Part model, mm, in its own coordinate system. A direction names the side the tool comes from. Give positions to 0.01 mm unless a question says otherwise; leave off trailing zeros. Loops run counter-clockwise (first coordinate to the right, second up) from the corner with the lowest first, then second, coordinate; pieces in that order, holes last. Notation, with made-up numbers: (-6, 50) -> (7, 50) arc R17 ccw to (7, 57) -> close; hole circle Ø9 at (-5.75, -27.75). An arc over 180 degrees is marked (long way). Write item = value, one per line.
from build123d import *

# Parameters (mm, degrees)
SKETCH1_W               = 12
SKETCH1_H               = 12
SKETCH1_R               = 5.5
BOSS_EXTRUDE1_DEPTH     = 6
BOSS_EXTRUDE1_2_DEPTH   = 6
BOSS_EXTRUDE1_3_DEPTH   = 6
BOSS_EXTRUDE1_4_DEPTH   = 6
BOSS_EXTRUDE1_5_DEPTH   = 6
BOSS_EXTRUDE1_6_DEPTH   = 6
BOSS_EXTRUDE2_START     = -6
BOSS_EXTRUDE2_OUTLINE_R = 1.7
BOSS_EXTRUDE2_DEPTH     = 6
CUT_EXTRUDE1_DEPTH      = 1


# Read off the part's stored shape, not the designer's step: Boss-Extrude2
with BuildPart() as part:
    # Sketch1 → Boss-Extrude1 (new body)
    with BuildSketch(Plane(origin=(0, 0, 0), x_dir=(1, 0, 0), z_dir=(0, 1, 0))):
        with Locations((13.686388819, -10.664882883)):
            Rectangle(SKETCH1_W, SKETCH1_H)
        with Locations(Location((13.686388819, -10.664882883, 0), (0, 0, 270))):
            Circle(SKETCH1_R, mode=Mode.SUBTRACT)
    extrude(amount=-BOSS_EXTRUDE1_DEPTH)



with BuildPart() as body_2:
    # Sketch1 → Boss-Extrude1 2 (new body)
    with BuildSketch(Plane(origin=(0, 0, 0), x_dir=(1, 0, 0), z_dir=(0, 1, 0))):
        with Locations((-1.113611181, -10.664882883)):
            Rectangle(SKETCH1_W, SKETCH1_H)
        with Locations(Location((-1.113611181, -10.664882883, 0), (0, 0, 270))):
            Circle(SKETCH1_R, mode=Mode.SUBTRACT)
    extrude(amount=-BOSS_EXTRUDE1_2_DEPTH)


with BuildPart() as body_3:
    # Sketch1 → Boss-Extrude1 3 (new body)
    with BuildSketch(Plane(origin=(0, 0, 0), x_dir=(1, 0, 0), z_dir=(0, 1, 0))):
        with Locations((6.28638882, -23.664882883)):
            Rectangle(SKETCH1_W, SKETCH1_H)
        with Locations(Location((6.28638882, -23.664882883, 0), (0, 0, 270))):
            Circle(SKETCH1_R, mode=Mode.SUBTRACT)
    extrude(amount=-BOSS_EXTRUDE1_3_DEPTH)


with BuildPart() as body_4:
    # Sketch1 → Boss-Extrude1 4 (new body)
    with BuildSketch(Plane(origin=(0, 0, 0), x_dir=(1, 0, 0), z_dir=(0, 1, 0))):
        with Locations((21.08638882, -23.664882883)):
            Rectangle(SKETCH1_W, SKETCH1_H)
        with Locations(Location((21.08638882, -23.664882883, 0), (0, 0, 270))):
            Circle(SKETCH1_R, mode=Mode.SUBTRACT)
    extrude(amount=-BOSS_EXTRUDE1_4_DEPTH)


with BuildPart() as body_5:
    # Sketch1 → Boss-Extrude1 5 (new body)
    with BuildSketch(Plane(origin=(0, 0, 0), x_dir=(1, 0, 0), z_dir=(0, 1, 0))):
        with Locations((35.88638882, -23.664882883)):
            Rectangle(SKETCH1_W, SKETCH1_H)
        with Locations(Location((35.88638882, -23.664882883, 0), (0, 0, 270))):
            Circle(SKETCH1_R, mode=Mode.SUBTRACT)
    extrude(amount=-BOSS_EXTRUDE1_5_DEPTH)


with BuildPart() as body_6:
    # Sketch1 → Boss-Extrude1 6 (new body)
    with BuildSketch(Plane(origin=(0, 0, 0), x_dir=(1, 0, 0), z_dir=(0, 1, 0))):
        with Locations((28.486388819, -10.664882883)):
            Rectangle(SKETCH1_W, SKETCH1_H)
        with Locations(Location((28.486388819, -10.664882883, 0), (0, 0, 270))):
            Circle(SKETCH1_R, mode=Mode.SUBTRACT)
    extrude(amount=-BOSS_EXTRUDE1_6_DEPTH)


with BuildPart() as part_1:
    add(part.part)

    add(body_2.part)  # Boss-Extrude2 merges body 2

    add(body_3.part)  # Boss-Extrude2 merges body 3

    add(body_4.part)  # Boss-Extrude2 merges body 4

    add(body_5.part)  # Boss-Extrude2 merges body 5

    add(body_6.part)  # Boss-Extrude2 merges body 6
    # Boss-Extrude2 outline → Boss-Extrude2 (add)
    with BuildSketch(Plane(origin=(0, 0, 0), x_dir=(1, 0, 0), z_dir=(0, 1, 0)).offset(BOSS_EXTRUDE2_START)):
        Polygon((11.186388819, -4.164882883), (1.386388819, -4.164882883), (1.386388819, -4.664882883), (4.886388819, -4.664882883), (4.886388819, -16.664882883), (-7.113611181, -16.664882883), (-7.113611181, -4.664882883), (-3.613611181, -4.664882883), (-3.613611181, -4.164882883), (-18.613611181, -4.164883527), (-18.613611181, -30.164882449), (3.78638882, -30.164882883), (3.78638882, -29.664882883), (0.28638882, -29.664882883), (0.28638882, -17.664882883), (12.28638882, -17.664882883), (12.28638882, -29.664882883), (8.78638882, -29.664882883), (8.78638882, -30.164882883), (18.58638882, -30.164882883), (18.58638882, -29.664882883), (15.08638882, -29.664882883), (15.08638882, -17.664882883), (27.08638882, -17.664882883), (27.08638882, -29.664882883), (23.58638882, -29.664882883), (23.58638882, -30.164882883), (33.38638882, -30.164882883), (33.38638882, -29.664882883), (29.88638882, -29.664882883), (29.88638882, -17.664882883), (41.88638882, -17.664882883), (41.88638882, -29.664882883), (38.38638882, -29.664882883), (38.38638882, -30.164882883), (53.38638882, -30.164882883), (53.38638882, -4.164882883), (30.986388819, -4.164882883), (30.986388819, -4.664882883), (34.486388819, -4.664882883), (34.486388819, -16.664882883), (22.486388819, -16.664882883), (22.486388819, -4.664882883), (25.986388819, -4.664882883), (25.986388819, -4.164882883), (16.186388819, -4.164882883), (16.186388819, -4.664882883), (19.686388819, -4.664882883), (19.686388819, -16.664882883), (7.686388819, -16.664882883), (7.686388819, -4.664882883), (11.186388819, -4.664882883), align=None)
        with Locations((-13.613611181, -17.164882988)):
            Circle(BOSS_EXTRUDE2_OUTLINE_R, mode=Mode.SUBTRACT)
        with Locations((48.386388819, -17.164882988)):
            Circle(BOSS_EXTRUDE2_OUTLINE_R, mode=Mode.SUBTRACT)
    extrude(amount=BOSS_EXTRUDE2_DEPTH)

    # Sketch2 → Cut-Extrude1 (cut)
    with BuildSketch(Plane.XZ.offset(6)):
        Polygon((-11.090813446, 25.393846705), (-9.544018575, 25.393846705), (-9.544018575, 25.068205679), (-10.805877549, 25.068205679), (-10.805877549, 24.091282602), (-9.544018575, 24.091282602), (-9.544018575, 23.765641577), (-10.805877549, 23.765641577), (-10.805877549, 22.218846705), (-11.090813446, 22.218846705), align=None)
        with BuildLine():
            Line((-8.852031395, 24.416923628), (-9.136967293, 24.416923628))
            add(Edge.make_bspline(
                [(-9.136967293, 24.416923628), (-9.135110232, 24.454725076), (-9.131463015, 24.528966114), (-9.114383067, 24.637209944), (-9.089943843, 24.74067394), (-9.055389453, 24.838527362), (-9.012475901, 24.931635423), (-8.961013662, 25.019628294), (-8.90005924, 25.102170301), (-8.830928846, 25.178496252), (-8.755845866, 25.248516405), (-8.674832621, 25.308982233), (-8.589701775, 25.360070406), (-8.500711605, 25.402779818), (-8.406858094, 25.434838107), (-8.30899293, 25.45862488), (-8.206686142, 25.472936279), (-8.136981265, 25.474474599), (-8.101530594, 25.475256961)],
                knots=[0, 0, 0, 0, 1.10065271, 2.161652631, 3.183658789, 4.190468796, 5.17591951, 6.163126047, 7.15150782, 8.156236427, 9.156009102, 10.134482811, 11.092018607, 12.041330605, 13.001268258, 13.972401359, 14.968799086, 16, 16, 16, 16], degree=3))
            add(Edge.make_bspline(
                [(-8.101530594, 25.475256961), (-8.066716198, 25.474441933), (-7.998307154, 25.472840431), (-7.898465184, 25.459087212), (-7.803417209, 25.437546568), (-7.713349021, 25.407324726), (-7.628979234, 25.366698853), (-7.549674044, 25.3178968), (-7.474489308, 25.261454524), (-7.406810297, 25.195002851), (-7.344663683, 25.124062116), (-7.291049494, 25.048326661), (-7.245136124, 24.97010438), (-7.206865872, 24.888798797), (-7.178693517, 24.803644364), (-7.157304714, 24.71588083), (-7.145214846, 24.624599752), (-7.143359355, 24.562817376), (-7.142416011, 24.531406801)],
                knots=[0, 0, 0, 0, 1.111607364, 2.184268762, 3.212621178, 4.221274766, 5.211760367, 6.196651075, 7.1921475, 8.207485113, 9.220403448, 10.201281604, 11.166441695, 12.114753415, 13.065576456, 14.026450734, 14.996634279, 16, 16, 16, 16], degree=3))
            add(Edge.make_bspline(
                [(-7.142416011, 24.531406801), (-7.143946038, 24.48718376), (-7.146979244, 24.399513729), (-7.173155489, 24.270514062), (-7.21359782, 24.145414473), (-7.262649782, 24.044740618), (-7.31219844, 23.964025865), (-7.355904397, 23.896973819), (-7.408203317, 23.825466998), (-7.468616685, 23.748785207), (-7.536233124, 23.666693885), (-7.611539287, 23.579159348), (-7.695110449, 23.487111285), (-7.753764656, 23.424241012), (-7.784157797, 23.391663211)],
                knots=[0, 0, 0, 0, 1.184203166, 2.347625244, 3.513805382, 4.700623107, 5.337941753, 6.051866363, 6.845199593, 7.711357327, 8.668078039, 9.695487809, 10.805859518, 12, 12, 12, 12], degree=3))
            Line((-7.784157797, 23.391663211), (-8.578543815, 22.544487731))
            Line((-8.578543815, 22.544487731), (-7.101710882, 22.544487731))
            Line((-7.101710882, 22.544487731), (-7.101710882, 22.218846705))
            Line((-7.101710882, 22.218846705), (-9.259082677, 22.218846705))
            Line((-9.259082677, 22.218846705), (-8.027752549, 23.532859125))
            add(Edge.make_bspline(
                [(-8.027752549, 23.532859125), (-7.997773395, 23.564154017), (-7.940189574, 23.624265101), (-7.858743951, 23.712024786), (-7.785592869, 23.793440441), (-7.720262805, 23.868358238), (-7.664170983, 23.937874018), (-7.614394029, 23.999736356), (-7.574510957, 24.056663607), (-7.531226277, 24.122649736), (-7.489303594, 24.203215195), (-7.453278814, 24.301670756), (-7.431312487, 24.403023335), (-7.428677386, 24.471514469), (-7.427351908, 24.505966096)],
                knots=[0, 0, 0, 0, 1.329631726, 2.553950428, 3.673215718, 4.687767853, 5.603093632, 6.413772471, 7.123043292, 7.734684054, 8.834405432, 9.900288307, 10.943827018, 12, 12, 12, 12], degree=3))
            add(Edge.make_bspline(
                [(-7.427351908, 24.505966096), (-7.427928617, 24.527629936), (-7.4290652, 24.570325205), (-7.439096111, 24.632923286), (-7.454254927, 24.693307081), (-7.475976697, 24.751662329), (-7.504648526, 24.807402313), (-7.539549378, 24.860594884), (-7.579817506, 24.912019874), (-7.626400444, 24.960237509), (-7.677573751, 25.004398317), (-7.731634249, 25.043518023), (-7.7888297, 25.076210645), (-7.848918954, 25.103010817), (-7.911734487, 25.124034199), (-7.977397792, 25.138601624), (-8.045727435, 25.147747878), (-8.092384963, 25.148985376), (-8.116158999, 25.149615936)],
                knots=[0, 0, 0, 0, 0.991446411, 1.95395049, 2.89581595, 3.838931463, 4.798493298, 5.75982156, 6.748411868, 7.785213223, 8.824556874, 9.840280684, 10.836137867, 11.835679398, 12.848801643, 13.863922112, 14.911575587, 16, 16, 16, 16], degree=3))
            add(Edge.make_bspline(
                [(-8.116158999, 25.149615936), (-8.140988255, 25.148967299), (-8.189748813, 25.147693485), (-8.26133965, 25.138782925), (-8.329634605, 25.123410627), (-8.394805474, 25.102386072), (-8.456962527, 25.07566296), (-8.515803481, 25.042378306), (-8.571196245, 25.002660423), (-8.623244948, 24.957629347), (-8.671200129, 24.907493737), (-8.713334081, 24.851604699), (-8.75014958, 24.790982687), (-8.782270813, 24.725791273), (-8.808356332, 24.655438916), (-8.828289118, 24.580175355), (-8.844061472, 24.500327387), (-8.84933063, 24.445186632), (-8.852031395, 24.416923628)],
                knots=[0, 0, 0, 0, 1.031018746, 2.02475058, 2.990194455, 3.934040569, 4.864654155, 5.795059489, 6.735614925, 7.690564532, 8.649604399, 9.611025574, 10.590972636, 11.591080095, 12.624614302, 13.701020113, 14.821632451, 16, 16, 16, 16], degree=3))
        make_face()
    extrude(amount=-CUT_EXTRUDE1_DEPTH, mode=Mode.SUBTRACT)


solid = part_1.part
1) Pull direction X, two halves, no side cores. Call faces 1 (the face through (-1, -3, 4.665)), 2 (the face through (46, -3, 30.165)), 3 (the face through (6, -3, 29.665)): pulls with the +X half, pulls with the -X half, needs draft (parallel to the pull), parting line crosses it, or undercut.
Resolved:
face_1 = undercut
face_2 = needs draft
face_3 = undercut
2) Which spindle directions (+Z, -Z, +X, -X, +Y, -Y) get a long thin tool onto all of the face, cutting with end or side? Do faces 4 (the face through (-15.31, -3.04, 17.09)), 5 (the face through (28, -3, 4.665)), 6 (the face through (21, -3, 29.665)). Say none if no direction does.
Resolved:
face_4 = +Y, -Y
face_5 = -Z, +Y, -Y
face_6 = +Z, +Y, -Y
3) Slice it at C-C, the plane x = 9.5. List the corners of the cut face in (y, z), and give its area (3 significant figures).
Resolved:
outline = (-6, 4.16) -> (0, 4.16) -> (0, 7.1) -> (-6, 7.1) -> close; (-6, 14.23) -> (0, 14.23) -> (0, 19.2) -> (-6, 19.2) -> close; (-6, 28.13) -> (0, 28.13) -> (0, 30.16) -> (-6, 30.16) -> close
area = 59.6 mm²
4) Drop flat-ended pins along their axis: P1, Ø1.5, axis at x = 20.5, y = -4, coming from the +Z side; P2, Ø6.5, axis at x = 6.29, z = 23.66, coming from the +Y side. Give the stop position or say it passes through.
Resolved:
P1 = 29.66
P2 = through
5) Slice it at A-A, the plane x = 27.5. List the corners of the cut face in (y, z).
Resolved:
outline = (-6, 4.66) -> (0, 4.66) -> (0, 5.25) -> (-6, 5.25) -> close; (-6, 16.08) -> (0, 16.08) -> (0, 30.16) -> (-6, 30.16) -> close
6) Slice it at B-B, the plane z = 10. List the corners of the cut face in (x, y), and give its area (3 significant figures).
Resolved:
outline = (-18.61, -6) -> (-6.57, -6) -> (-6.57, 0) -> (-18.61, 0) -> close; (4.35, -6) -> (8.23, -6) -> (8.23, 0) -> (4.35, 0) -> close; (19.15, -6) -> (23.03, -6) -> (23.03, 0) -> (19.15, 0) -> close; (33.95, -6) -> (53.39, -6) -> (53.39, 0) -> (33.95, 0) -> close
area = 235 mm²
7) Drill centre lines: line 1 along X through (y, z) = (-5, 10.5); line 2 along Z through (x, y) = (-1, -0.25); line 3 along X through (y, z) = (-3.25, 27.25). Where is each one in solid material? Low to high. Write a range as [from, to].
Resolved:
line_1 = [-18.61, -6.61], [4.38, 8.19], [19.18, 22.99], [33.98, 53.39]
line_2 = [4.66, 5.17], [16.16, 30.16]
line_3 = [-18.61, 2.12], [10.46, 16.92], [25.26, 31.72], [40.06, 53.39]
8) Slice it at D-D, the plane y = -1.75. Count the separate pieces of the cut face and the enclosed holes in it, and give its area (3 significant figures).
Resolved:
separate_pieces = 1
enclosed_holes = 8
area = 1,270 mm²
